The figure shows three views and two pictorial views of one solid part (mm, origin at its lowest corner). Answer the questions. Coordinates: 2 decimals unless noted, no trailing zeros. Write each loop counter-clockwise with the first axis right and the second up, starting at its lowest first coordinate (ties: lowest second). Pieces come first, ordered by that corner, then holes.
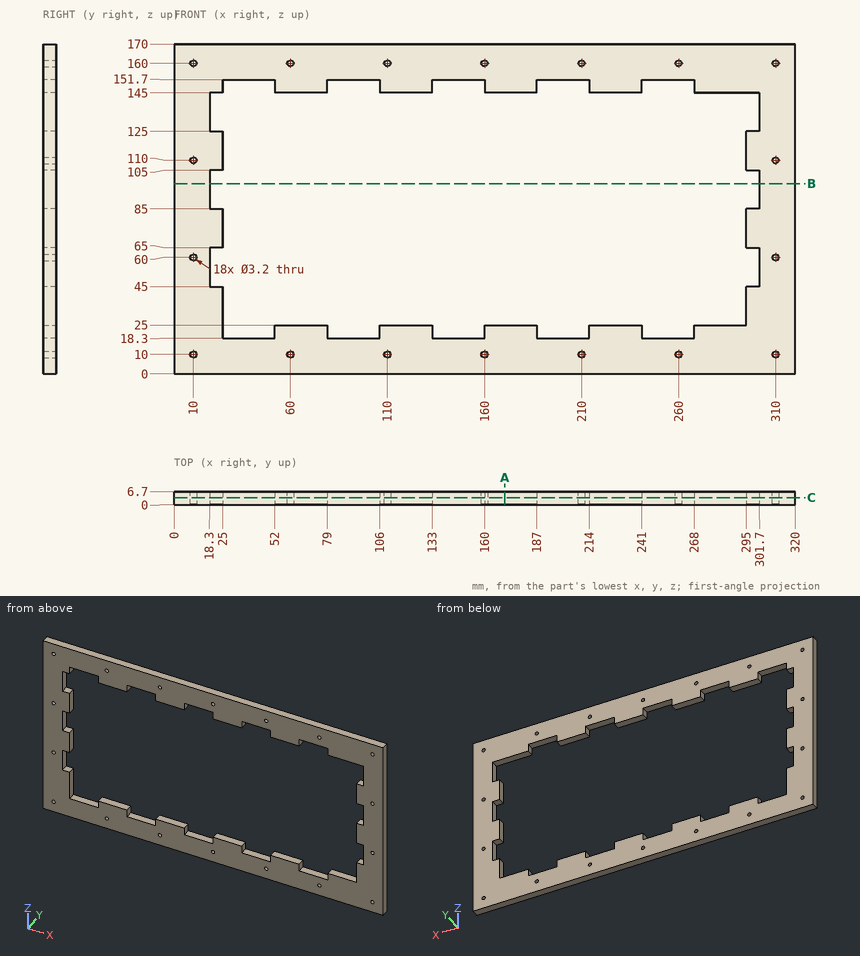
1. Section A-A on x = 170.5 is taken. Give the vertices of the cut face in (y, z).
Results found:
outline: (0, 0) - (6.7, 0) - (6.7, 25) - (0, 25) - close; (0, 145) - (6.7, 145) - (6.7, 170) - (0, 170) - close
2. Find the intervals of material crossed by L1, parallel to Z at x = 10, y = 1.75; L2, parallel to Z at x = 260, y = 3; L3, parallel to X at y = 1.5, z = 18.5, in increasing order.
Results found:
L1: z = 0 to 8.4, 11.6 to 58.4, 61.6 to 108.4, 111.6 to 158.4, 161.6 to 170
L2: z = 0 to 8.4, 11.6 to 18.3, 151.7 to 158.4, 161.6 to 170
L3: x = 0 to 25, 52 to 79, 106 to 133, 160 to 187, 214 to 241, 268 to 320
3. Section B-B on z = 98 is taken. Give the vertices of the cut face in (x, y).
Results found:
outline: (0, 0) - (18.3, 0) - (18.3, 6.7) - (0, 6.7) - close; (301.7, 0) - (320, 0) - (320, 6.7) - (301.7, 6.7) - close
4. Section C-C on y = 3.75 is taken. State how many separate pieces and enclosed holes the cut face has, then the cut area to 3 significant figures.
Results found:
separate pieces: 1
enclosed holes: 19
area: 19,200 mm2
